Input: part model. Units: mm. Frame: model coordinates. A direction names the side the tool comes from. Round coordinates to 2 decimals unless told otherwise and drop trailing zeros. Order: outer loops, then holes, each group sorted by start corner. A loop starts at its lowest first (then second) coordinate and runs counter-clockwise, first axis right, second up. Notation, with made-up numbers: (80, 12) -> (84, 12) arc R23 cw to (84, 48) -> close; hole circle Ø1 at (59.5, 60.5). An arc over 180 degrees is marked (long way). Answer as CSV lines item,"result". Start each with the question number.
1) Line query: L1, parallel to Z at x = -181, y = 68.5; L2, parallel to X at y = 39, z = -152; L3, parallel to Y at x = -163, z = -23. Output: solid intervals per line, ascending.
2) Mould query, pull axis Y, two halves, no side actions, for faces 4 (the face through (-196.58, 75.5, -84.16)), 5 (the face through (-172, 51, -163)), 6 (the face through (-172, 51, -3)), 7 (the face through (-178, 57, -166)). Classes: +Y half, -Y half, draft (parallel to the pull), parting line (faces both ways), or undercut.
3) Section query D-D, the plane z = -154. Output: boundary loops of the cut face in (x, y), and give its area (3 significant figures).
4) Access query for faces 1 (the face through (-194.504, 73.574, -84.12)), 2 (the face through (-154, 43, -1)), 3 (the face through (-187.28, 76.01, -123.03)). Directions: +Z, -Z, +X, -X, +Y, -Y. A direction counts if a zero-diameter tool reaches every point of the face in a straight line with its end or side. Return the directions, or none.
5) Section query A-A, the plane z = -109. State how many separate pieces and enclosed holes the cut face has, and give its area (3 significant figures).
6) Section query C-C, the plane x = -156. Output: boundary loops of the cut face in (y, z).
7) Section query B-B, the plane z = -60. Output: boundary loops of the cut face in (x, y).
8) First-contact query: P1, Ø2, axis at x = -197, z = -75, coming from the -Y side; P2, Ø1, axis at x = -197, z = -90, coming from the +Y side; P3, Ø2, axis at y = 36.5, z = -136, coming from the +X side; P4, Ø1.1, axis at x = -197.5, y = 65.5, coming from the +Z side. Flat tips, straight axial feed; report the tip coordinate or a pass-through.
```python
from build123d import *

# Parameters (mm, degrees)
BOSS_EXTRUDE1_DEPTH = 3
BOSS_EXTRUDE2_DEPTH = 3
BOSS_EXTRUDE3_DEPTH = 160
FILLET1_R           = 5
FILLET2_R           = 25
CUT_EXTRUDE1_DEPTH  = 5
SKETCH5_R           = 8
CUT_EXTRUDE2_DEPTH  = 2
SKETCH6_R           = 1.6
CUT_EXTRUDE3_DEPTH  = 2
SKETCH7_R           = 5
CUT_EXTRUDE4_DEPTH  = 3


with BuildPart() as part:
    # Sketch1 → Boss-Extrude1 (new body)
    with BuildSketch(Plane.XY):
        with BuildLine():
            Line((-176.422637822, 3.646230224), (-198.007283518, 24.991807553))
            Line((-198.007283518, 24.991807553), (-198.007283518, 77))
            Line((-198.007283518, 77), (-148.007283518, 77))
            Line((-148.007283518, 77), (-148.007283518, 43))
            Line((-148.007283518, 43), (-160.25, 43))
            ThreePointArc((-160.25, 43), (-181.523653951, 28.742519521), (-176.422637822, 3.646230224))
        make_face()
    extrude(amount=-BOSS_EXTRUDE1_DEPTH)



with BuildPart() as body_2:
    # Sketch2 → Boss-Extrude2 (new body)
    with BuildSketch(Plane(origin=(0, 0, -166), x_dir=(-1, 0, 0), z_dir=(0, 0, -1))):
        with BuildLine():
            Line((198.007283518, 24.991807553), (198.007283518, 77))
            Line((198.007283518, 77), (148.007283518, 77))
            Line((148.007283518, 77), (148.007283518, 43))
            Line((148.007283518, 43), (160.25, 43))
            ThreePointArc((160.25, 43), (181.523653951, 28.742519521), (176.422637822, 3.646230224))
            Line((176.422637822, 3.646230224), (198.007283518, 24.991807553))
        make_face()
    extrude(amount=-BOSS_EXTRUDE2_DEPTH)


with BuildPart() as part_1:
    add(part.part)

    add(body_2.part)  # Boss-Extrude3 merges body 2
    # Sketch3 → Boss-Extrude3 (add)
    with BuildSketch(Plane(origin=(0, 0, -3), x_dir=(-1, 0, 0), z_dir=(0, 0, -1))):
        with BuildLine():
            Line((181.686406663, 11.66450545), (196.007283518, 25.826766376))
            Line((196.007283518, 25.826766376), (196.007283518, 75))
            Line((196.007283518, 75), (148.007283518, 75))
            Line((148.007283518, 75), (148.007283518, 77))
            Line((148.007283518, 77), (198.007283518, 77))
            Line((198.007283518, 77), (198.007283518, 24.991807553))
            Line((198.007283518, 24.991807553), (176.422637822, 3.646230224))
            ThreePointArc((176.422637822, 3.646230224), (179.477148545, 7.377925731), (181.686406663, 11.66450545))
        make_face()
    extrude(amount=BOSS_EXTRUDE3_DEPTH)

    # Fillet1
    fillet1_edges = [part_1.edges().sort_by_distance(p)[0] for p in [
        (-198.007283518, 77, -83),
        (-196.007283518, 75, -83),
    ]]
    fillet(fillet1_edges, radius=FILLET1_R)

    # Fillet2
    fillet2_edges = [part_1.edges().sort_by_distance(p)[0] for p in [
        (-198.007283518, 24.991807553, -83),
        (-196.007283518, 25.826766376, -83),
    ]]
    fillet(fillet2_edges, radius=FILLET2_R)

    # Sketch4 → Cut-Extrude1 (cut)
    with BuildSketch(Plane.ZY.offset(198.007283518)):
        with BuildLine():
            Line((-112, 59.5), (-54, 59.5))
            ThreePointArc((-54, 59.5), (-53.292893219, 59.207106781), (-53, 58.5))
            Line((-53, 58.5), (-53, 57.5))
            ThreePointArc((-53, 57.5), (-53.292893219, 56.792893219), (-54, 56.5))
            Line((-54, 56.5), (-112, 56.5))
            ThreePointArc((-112, 56.5), (-112.707106781, 56.792893219), (-113, 57.5))
            Line((-113, 57.5), (-113, 58.5))
            ThreePointArc((-113, 58.5), (-112.707106781, 59.207106781), (-112, 59.5))
        make_face()
        with BuildLine():
            Line((-112, 67), (-54, 67))
            ThreePointArc((-54, 67), (-53.292893219, 66.707106781), (-53, 66))
            Line((-53, 66), (-53, 65))
            ThreePointArc((-53, 65), (-53.292893219, 64.292893219), (-54, 64))
            Line((-54, 64), (-112, 64))
            ThreePointArc((-112, 64), (-112.707106781, 64.292893219), (-113, 65))
            Line((-113, 65), (-113, 66))
            ThreePointArc((-113, 66), (-112.707106781, 66.707106781), (-112, 67))
        make_face()
        with BuildLine():
            Line((-112, 52), (-54, 52))
            ThreePointArc((-54, 52), (-53.292893219, 51.707106781), (-53, 51))
            Line((-53, 51), (-53, 50))
            ThreePointArc((-53, 50), (-53.292893219, 49.292893219), (-54, 49))
            Line((-54, 49), (-112, 49))
            ThreePointArc((-112, 49), (-112.707106781, 49.292893219), (-113, 50))
            Line((-113, 50), (-113, 51))
            ThreePointArc((-113, 51), (-112.707106781, 51.707106781), (-112, 52))
        make_face()
        with BuildLine():
            Line((-112, 44.5), (-54, 44.5))
            ThreePointArc((-54, 44.5), (-53.292893219, 44.207106781), (-53, 43.5))
            Line((-53, 43.5), (-53, 42.5))
            ThreePointArc((-53, 42.5), (-53.292893219, 41.792893219), (-54, 41.5))
            Line((-54, 41.5), (-112, 41.5))
            ThreePointArc((-112, 41.5), (-112.707106781, 41.792893219), (-113, 42.5))
            Line((-113, 42.5), (-113, 43.5))
            ThreePointArc((-113, 43.5), (-112.707106781, 44.207106781), (-112, 44.5))
        make_face()
    extrude(amount=-CUT_EXTRUDE1_DEPTH, mode=Mode.SUBTRACT)

    # Sketch5 → Cut-Extrude2 (cut)
    with BuildSketch(Plane(origin=(0, 77, 0), x_dir=(1, 0, 0), z_dir=(0, 1, 0))):
        with Locations((-170.507283518, 109)):
            Circle(SKETCH5_R)
    extrude(amount=-CUT_EXTRUDE2_DEPTH, mode=Mode.SUBTRACT)

    # Sketch6 → Cut-Extrude3 (cut)
    with BuildSketch(Plane(origin=(0, 77, 0), x_dir=(1, 0, 0), z_dir=(0, 1, 0))):
        with Locations((-156.007283518, 154)):
            Circle(SKETCH6_R)
        with Locations((-156.007283518, 124)):
            Circle(SKETCH6_R)
        with Locations((-186.007283518, 124)):
            Circle(SKETCH6_R)
        with Locations((-186.007283518, 154)):
            Circle(SKETCH6_R)
    extrude(amount=-CUT_EXTRUDE3_DEPTH, mode=Mode.SUBTRACT)

    # Sketch7 → Cut-Extrude4 (cut)
    with BuildSketch(Plane.ZY.offset(198.007283518)):
        with Locations((-141, 57)):
            Circle(SKETCH7_R)
    extrude(amount=-CUT_EXTRUDE4_DEPTH, mode=Mode.SUBTRACT)


solid = part_1.part
```
Findings:
1,L1,"z = -166 to -163, -3 to 0"
1,L2,"x = -198.01 to -196.01"
1,L3,"y = 75 to 77"
2,face 4,"+Y half"
2,face 5,"undercut"
2,face 6,"undercut"
2,face 7,"draft"
3,outline,"(-198.01, 35.43) arc R25 ccw to (-190.59, 17.65) -> (-176.42, 3.65) arc R23 cw to (-181.69, 11.66) -> (-188.59, 18.49) arc R25 cw to (-196.01, 36.26) -> (-196.01, 70) arc R5 cw to (-191.01, 75) -> (-187.61, 75) -> (-187.61, 77) -> (-193.01, 77) arc R5 ccw to (-198.01, 72) -> close; (-184.41, 75) -> (-157.61, 75) -> (-157.61, 77) -> (-184.41, 77) -> close; (-154.41, 75) -> (-148.01, 75) -> (-148.01, 77) -> (-154.41, 77) -> close"
3,area,"234 mm^2"
4,face 1,"+X"
4,face 2,"+Z, -Z, +X, -Y"
4,face 3,"+Y"
5,separate pieces,"6"
5,enclosed holes,"0"
5,area,"190 mm^2"
6,outline,"(43, -166) -> (77, -166) -> (77, -155.6) -> (75, -155.6) -> (75, -163) -> (43, -163) -> close; (43, -3) -> (75, -3) -> (75, -122.4) -> (77, -122.4) -> (77, 0) -> (43, 0) -> close; (75, -152.4) -> (77, -152.4) -> (77, -125.6) -> (75, -125.6) -> close"
7,outline,"(-198.01, 35.43) arc R25 ccw to (-190.59, 17.65) -> (-176.42, 3.65) arc R23 cw to (-181.69, 11.66) -> (-188.59, 18.49) arc R25 cw to (-196.01, 36.26) -> (-196.01, 41.5) -> (-198.01, 41.5) -> close; (-198.01, 44.5) -> (-196.01, 44.5) -> (-196.01, 49) -> (-198.01, 49) -> close; (-198.01, 52) -> (-196.01, 52) -> (-196.01, 56.5) -> (-198.01, 56.5) -> close; (-198.01, 59.5) -> (-196.01, 59.5) -> (-196.01, 64) -> (-198.01, 64) -> close; (-198.01, 67) -> (-196.01, 67) -> (-196.01, 70) arc R5 cw to (-191.01, 75) -> (-148.01, 75) -> (-148.01, 77) -> (-193.01, 77) arc R5 ccw to (-198.01, 72) -> close"
8,P1,"stops at y = 25.61"
8,P2,"stops at y = 75.58"
8,P3,"stops at x = -196"
8,P4,"stops at z = 0"
